Design review of the part built by this model. Coordinates are the model's own, in mm. A direction names the side the tool comes from. Round coordinates to 2 decimals unless told otherwise and drop trailing zeros. Write each loop counter-clockwise with the first axis right and the second up, starting at its lowest first coordinate (ties: lowest second). Pieces come first, ordered by that corner, then holes. Notation, with made-up numbers: (9.25, -3.75) - (43.25, -3.75) arc R29 cw to (43.25, 28.25) - close; hole circle Ø8 at (43.25, 67.5). An arc over 180 degrees is marked (long way). Use one line per item in the form item = value.
```python
from build123d import *

# Parameters (mm, degrees)
F0_R     = 12.7
F0_R_2   = 8.73125
F1_DEPTH = 3.175
F2_R     = 8.73125
F3_DEPTH = 9.525
F5_D     = 12.7


with BuildPart() as f1:
    # F0 (on Front) → F1 (new body)
    with BuildSketch(Plane.XZ):
        Circle(F0_R)
        Circle(F0_R_2, mode=Mode.SUBTRACT)
        Circle(F0_R_2)
    extrude(amount=F1_DEPTH)

    # F2 (on face) → F3 (join)
    with BuildSketch(Plane.XZ.offset(3.175)):
        Circle(F2_R)
    extrude(amount=F3_DEPTH)

    # F5 (through all)
    with Locations(Plane.XZ.offset(12.7)):
        with Locations((0, 1.5875)):
            Hole(F5_D / 2)


solid = f1.part
```
Q1. We need section A-A on x = 0. Write out the cut boundary in (y, z) (1 decimal), then the cut area to 3 significant figures.
Calculated:
outline = (-12.7, -8.7) - (-3.2, -8.7) - (-3.2, -12.7) - (0, -12.7) - (0, -4.8) - (-12.7, -4.8) - close; (-12.7, 7.9) - (0, 7.9) - (0, 12.7) - (-3.2, 12.7) - (-3.2, 8.7) - (-12.7, 8.7) - close
area = 85.7 mm2
Q2. We need section C-C on z = -5.5. Write out the cut boundary in (x, y) (3 decimals), then the cut area to 3 significant figures.
Calculated:
outline = (-11.447, -3.175) - (-6.781, -3.175) - (-6.781, -12.7) - (6.781, -12.7) - (6.781, -3.175) - (11.447, -3.175) - (11.447, 0) - (-11.447, 0) - close
area = 202 mm2
Q3. We need section D-D on y = -6.5. Write out the cut boundary in (x, z).
Calculated:
outline = circle Ø17.46 at (0, 0); hole circle Ø12.7 at (0, 1.59)
Q4. To check wall thickness, follow line 1 along Z through (x, y) = (0, -8.75); line 2 along Y through (x, z) = (-2.75, 9) (3 decimals); line 3 along Z through (x, y) = (0, -3). State the ranges of each line that lie inside material, in increasing order. Write a range as from..to.
Calculated:
line_1 = -8.73..-4.76, 7.94..8.73
line_2 = -3.175..0
line_3 = -12.7..-4.76, 7.94..12.7
Q5. Draft analysis for pull direction Z (two halves, no side actions). For faces 1 (the cylindrical face through (0.827, -6.261, 7.883)), 2 (the cylindrical face through (-6.93, -7.87, -5.31)), 3 (the flat face through (0, 0, -5)), state which applies: released by +Z, released by -Z, zero draft, split by the parting line, or undercut.
Calculated:
face_1 = undercut
face_2 = split by the parting line
face_3 = zero draft
Q6. We need section B-B on z = 5.5. Write out the cut boundary in (x, y) (3 decimals).
Calculated:
outline = (-11.447, -3.175) - (-6.781, -3.175) - (-6.781, -12.7) - (-5.001, -12.7) - (-5.001, 0) - (-11.447, 0) - close; (5.001, -12.7) - (6.781, -12.7) - (6.781, -3.175) - (11.447, -3.175) - (11.447, 0) - (5.001, 0) - close
Q7. For P1, Ø6, axis at x = 5, y = -8.5, coming from the +Z side; P2, Ø2, axis at y = -6.5, z = 1, coming from the -X side; P3, Ø1.5, axis at y = -3.5, z = -4, coming from the -X side, all flat-tipped, find the tip position at first contact; note any pin that passes through.
Calculated:
P1 = 8.5
P2 = -8.73
P3 = -12.26
Q8. Machinability: for faces 4 (the flat face through (3, -3.175, 9)), 5 (the flat face through (0, -12.7, -6)), which of the approach directions +Z, -Z, +X, -X, +Y, -Y give a long, thin tool a straight path to every point of the face, cutting with its end or side? Answer none if there is none.
Calculated:
face_4 = -Y
face_5 = +Z, -Z, +X, -X, -Y
